Part model, mm, in its own coordinate system. A direction names the side the tool comes from. Round coordinates to 2 decimals unless told otherwise and drop trailing zeros. Loops run counter-clockwise (first coordinate to the right, second up) from the corner with the lowest first, then second, coordinate; pieces in that order, holes last.
(1) Cut at A-A on x = 35. List the corners of the cut face in (y, z).
(2) Cut at D-D on z = 2. List the corners of the cut face in (x, y), then the cut area to 3 significant figures.
(3) Cut at C-C on z = 0. Count the separate pieces of the cut face and the enclosed holes in it, then the cut area to 3 significant figures.
(4) Mould opens along Z. For faces 1 (the face through (40.5, -51.49, 0.07)), 2 (the face through (49.51, -32.51, 0.99)), 3 (the face through (36, -31.5, 1)), 4 (the face through (36, -51, 0)) say: +Z half, -Z half, draft (parallel to the pull), parting line (faces both ways), or undercut.
(5) Tool access for faces 5 (the face through (30, -33, 3)), 6 (the face through (43.339, -52.215, 4.699)), 7 (the face through (37, -33.5, 0)): list every direction of +Z, -Z, +X, -X, +Y, -Y with a clear straight run to the whole face (end or side of a thin tool).
(6) Probe probe 1 along Y at (x, z) = (31, 2); probe 2 along X at (y, z) = (-32.55, 0); probe 3 along Z at (x, y) = (35, -51.55). List the from-to ranges inside material, lowest first.
(7) Cut at B-B on y = -33. List the corners of the cut face in (x, z), then the cut area to 3 significant figures.
(8) Flat gauge pins, fed straight in: pin 1 (0.6 mm diameter, centred on x = 29.5, y = -32.5, fed in from +Z); pin 2 (1.6 mm diameter, centred on y = -45, z = 4.5, fed in from -X); pin 3 (8.5 mm diameter, centred on x = 49, y = -44.5, fed in from -Z). Where does each tip first touch, or does it go through?
from build123d import *

# Parameters (mm, degrees)
SKETCH002_R       = 1.5
SKETCH002_R_2     = 1
PAD002_DEPTH      = 10.5
SKETCH003_W       = 17
SKETCH003_H       = 9.673154
POCKET_DEPTH      = 27.001
POCKET_DEPTH_BACK = 3.001
FILLET002_R       = 1


with BuildPart() as part:
    # Sketch002 → Pad002 (new body, symmetric)
    with BuildSketch(Plane.XZ):
        with BuildLine():
            ThreePointArc((0, 3), (-3, 0), (0, -3))
            Line((0, -3), (17, -3))
            ThreePointArc((27, 3), (21.433882, 0.94353), (17, -3))
            Line((27, 3), (27, 5))
            Line((27, 5), (4, 5))
            Line((4, 5), (4, 3))
            Line((0, 3), (4, 3))
        make_face()
        Circle(SKETCH002_R, mode=Mode.SUBTRACT)
        with Locations((7, 0)):
            Circle(SKETCH002_R_2, mode=Mode.SUBTRACT)
        with Locations((14, 0)):
            Circle(SKETCH002_R, mode=Mode.SUBTRACT)
    extrude(amount=PAD002_DEPTH, both=True)

    # Sketch003 → Pocket (cut, two sides)
    with BuildSketch(Plane(origin=(0, 0, 0), x_dir=(0, -1, 0), z_dir=(-1, 0, 0))) as pocket_sk:
        with Locations((0, -1.836577)):
            Rectangle(SKETCH003_W, SKETCH003_H)
    extrude(amount=-POCKET_DEPTH, mode=Mode.SUBTRACT)
    extrude(pocket_sk.sketch, amount=POCKET_DEPTH_BACK, mode=Mode.SUBTRACT)

    # Fillet002
    fillet002_edges = [part.edges().sort_by_distance(p)[0] for p in [
        (15.5, 10.5, 5),
        (15.5, -10.5, 5),
    ]]
    fillet(fillet002_edges, radius=FILLET002_R)


with BuildPart() as part_1:
    # Body001 placement: moved
    add(part.part.moved(Location((28, -42, 0))))


solid = part_1.part
Final values:
1. outline: (-52.5, -3) - (-50.5, -3) - (-50.5, -1) - (-52.5, -1) - close; (-52.5, 1) - (-50.5, 1) - (-50.5, 3) - (-33.5, 3) - (-33.5, 1) - (-31.5, 1) - (-31.5, 4) arc R1 ccw to (-32.5, 5) - (-51.5, 5) arc R1 ccw to (-52.5, 4) - close; (-33.5, -3) - (-31.5, -3) - (-31.5, -1) - (-33.5, -1) - close
2. outline: (25.76, -52.5) - (51.53, -52.5) - (51.53, -50.5) - (25.76, -50.5) - close; (25.76, -33.5) - (51.53, -33.5) - (51.53, -31.5) - (25.76, -31.5) - close
2. area: 103 mm2
3. separate pieces: 8
3. enclosed holes: 0
3. area: 60.1 mm2
4. face 1: undercut
4. face 2: -Z half
4. face 3: draft
4. face 4: undercut
5. face 5: +Z, -X, +Y, -Y
5. face 6: +Z, +X, -X, -Y
5. face 7: -Z, +X, -X
6. probe 1: y = -52.5 to -50.5, -33.5 to -31.5
6. probe 2: x = 25 to 26.5, 29.5 to 34, 36 to 40.5, 43.5 to 48.03
6. probe 3: z = -3 to -1, 1 to 5
7. outline: (28, -3) - (45, -3) arc R16 cw to (55, 3) - (55, 5) - (32, 5) - (32, 3) - (28, 3) arc R3 ccw to start; hole circle Ø3 at (28, 0); hole circle Ø2 at (35, 0); hole circle Ø3 at (42, 0)
7. area: 166 mm2
8. pin 1: stops at z = 3
8. pin 2: stops at x = 32
8. pin 3: stops at z = 3
